Source: CAD feature listing. Evaluate the final solid. Frame: model axes, mm. Face numbers are marked on the shaded views. Give positions to 0.01 mm unless a question says otherwise; leave off trailing zeros. Write each loop counter-clockwise with the first axis right and the second up, starting at its lowest first coordinate (ties: lowest second). Pieces come first, ordered by that corner, then holes.
```python
from build123d import *

# Parameters (mm, degrees)
SKETCH_R           = 66.25
PAD_DEPTH          = 6
SKETCH001_R        = 5.5
POCKET_DEPTH       = 6.001
SKETCH002_R        = 2
POCKET001_DEPTH    = 380.959664
POLARPATTERN_COUNT = 3
CHAMFER_SIZE       = 1
FILLET_R           = 6
SKETCH003_R        = 64
POCKET002_DEPTH    = 3


with BuildPart() as part:
    # Sketch → Pad (new body)
    with BuildSketch(Plane.XY):
        Circle(SKETCH_R)
    extrude(amount=PAD_DEPTH)

    # Sketch001 → Pocket (cut, through all)
    with BuildSketch(Plane.XY):
        Circle(SKETCH001_R)
    extrude(amount=POCKET_DEPTH, mode=Mode.SUBTRACT)

    # Sketch002 → Pocket001 (cut, through all)
    with BuildSketch(Plane.XY):
        with Locations((0, 50)):
            Circle(SKETCH002_R)
        with BuildLine():
            ThreePointArc((-5, 59.791304), (-51.961524, 30), (-54.280788, -25.565525))
            Line((-10, 0), (-54.280788, -25.565525))
            ThreePointArc((-5, 8.660254), (-8.660254, 5), (-10, 0))
            Line((-5, 8.660254), (-5, 59.791304))
        make_face()
    pocket001 = extrude(amount=POCKET001_DEPTH, mode=Mode.SUBTRACT)

    # PolarPattern: Pocket001 ×3 about axis
    polarpattern_axis = Axis((0, 0, 0), (0, 0, 1))
    for i in range(1, POLARPATTERN_COUNT):
        add(pocket001.rotate(polarpattern_axis, i * 360 / POLARPATTERN_COUNT), mode=Mode.SUBTRACT)

    # Chamfer
    chamfer_edges = [part.edges().sort_by_distance(p)[0] for p in [
        (-66.25, 0, 6),
        (-66.25, 0, 0),
    ]]
    chamfer(chamfer_edges, length=CHAMFER_SIZE)

    # Fillet
    fillet_edges = [part.edges().sort_by_distance(p)[0] for p in [
        (-54.280788, -25.565525, 3),
        (-5, 59.791304, 3),
        (5, 59.791304, 3),
        (54.280788, -25.565525, 3),
        (49.280788, -34.225779, 3),
        (-49.280788, -34.225779, 3),
    ]]
    fillet(fillet_edges, radius=FILLET_R)

    # Sketch003 (on Face25 of Fillet) → Pocket002 (cut)
    with BuildSketch(Plane.XY.offset(6)):
        Circle(SKETCH003_R)
    extrude(amount=-POCKET002_DEPTH, mode=Mode.SUBTRACT)


solid = part.part
```
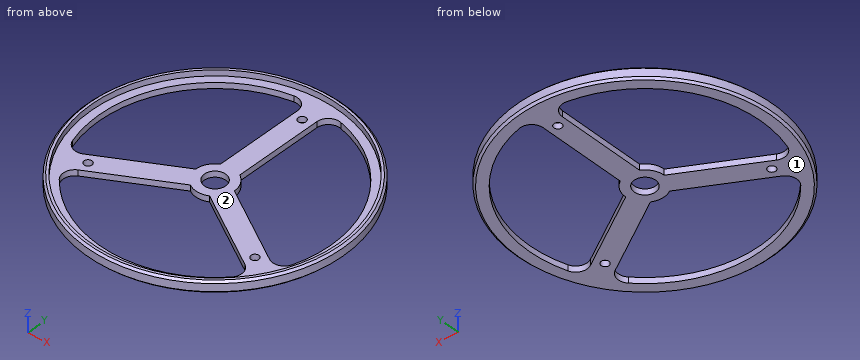
1. Cut plane C-C, the plane y = -25. State how many separate pieces and enclosed holes the cut face has, then the cut area to 3 significant figures.
2. Contact query for flat-ended pins moving along their axis: P1, Ø1, axis at y = 17.5, z = 5, coming from the +X side; P2, Ø1, axis at x = -47, z = 4.5, coming from the +Y side; P3, Ø6.5, axis at x = 0, y = 50, coming from the +Z side. Output: stop coordinate, or through.
3. Mould query, pull axis X, two halves, no side actions, for the marked faces 1 and 2. Classes: +X half, -X half, draft (parallel to the pull), parting line (faces both ways), or undercut.
4. Cut plane B-B, the plane z = 1.95. Return the cut outline in (x, y).
5. Cut plane A-A, the plane x = 0. Return the cut outline in (y, z).
6. Line query: L1, parallel to Y at x = 0, z = 2.4; L2, parallel to Y at x = 0, z = 4.35; L3, parallel to Y at x = 26, z = 0.8. Output: solid intervals per line, ascending.
Response values:
1. separate pieces: 4
1. enclosed holes: 0
1. area: 157 mm2
2. P1: stops at x = 64.03
2. P2: stops at y = 47.19
2. P3: stops at z = 3
3. face 1: draft
3. face 2: undercut
4. outline: circle Ø132.5 at (0, 0); hole (-56.98, -18.79) arc R6 ccw to (-48.28, -22.1) - (-10, 0) arc R10 cw to (-5, 8.66) - (-5, 52.87) arc R6 ccw to (-12.22, 58.74) arc R60 ccw to start; hole circle Ø4 at (-43.3, -25); hole (-44.76, -39.96) arc R60 ccw to (44.76, -39.96) arc R6 ccw to (43.28, -30.76) - (5, -8.66) arc R10 cw to (-5, -8.66) - (-43.28, -30.76) arc R6 ccw to start; hole circle Ø11 at (0, 0); hole circle Ø4 at (0, 50); hole (5, 8.66) arc R10 cw to (10, 0) - (48.28, -22.1) arc R6 ccw to (56.98, -18.79) arc R60 ccw to (12.22, 58.74) arc R6 ccw to (5, 52.87) - close; hole circle Ø4 at (43.3, -25)
5. outline: (-66.25, 1) - (-65.25, 0) - (-60, 0) - (-60, 3) - (-64, 3) - (-64, 6) - (-65.25, 6) - (-66.25, 5) - close; (-10, 0) - (-5.5, 0) - (-5.5, 3) - (-10, 3) - close; (5.5, 0) - (48, 0) - (48, 3) - (5.5, 3) - close; (52, 0) - (65.25, 0) - (66.25, 1) - (66.25, 5) - (65.25, 6) - (64, 6) - (64, 3) - (52, 3) - close
6. L1: y = -66.25 to -60, -10 to -5.5, 5.5 to 48, 52 to 66.25
6. L2: y = -66.25 to -64, 64 to 66.25
6. L3: y = -60.72 to -54.07, -20.78 to -9.24, 54.07 to 60.72
